Can you work these out from the model? Positions are in its coordinate system, mm. Face numbers are marked on the shaded views. A direction names the side the tool comes from. Give positions to 0.01 mm unless a question says otherwise; leave off trailing zeros. Loops run counter-clockwise (first coordinate to the right, second up) from the corner with the lowest first, then second, coordinate; pieces in that order, holes last. Notation, with made-up numbers: (25.25, -35) - (68.25, -35) arc R13 ccw to (68.25, -19) - close; hole circle Ø9 at (-27.5, 25). An arc over 180 degrees is marked (long way). Answer as a JSON object with one key per item and string values. Group by question number.
Item 1: Suppose I cut it at C-C on y = -0.75. Write out the boundary of the cut face in (x, z), and give its area (3 significant figures).
Item 2: Suppose I cut it at B-B on z = 9.5. Count the separate pieces of the cut face and the enclosed holes in it, and give its area (3 significant figures).
Item 3: Thinking about a two-plate mould opening in Y: for the marked faces 1, 2 and 3, which applies, pulls with the +Y half, pulls with the -Y half, needs draft (parallel to the pull), parting line crosses it, or undercut?
Item 4: Suppose I cut it at A-A on x = 0. Write out the boundary of the cut face in (y, z) (1 decimal).
Item 5: Which directions (+Z, -Z, +X, -X, +Y, -Y) give clear straight access to the entire face, cutting with the end or side of a thin tool? Please do the marked faces 4 and 5.
Item 6: Suppose I cut it at D-D on y = 12. Write out the boundary of the cut face in (x, z).
Item 7: Please list where these lines run through material, in increasing order: L1, parallel to Y at x = 0.25, z = 10; L2, parallel to X at y = 10.25, z = 8.25; L3, parallel to Y at x = 0, z = 8.
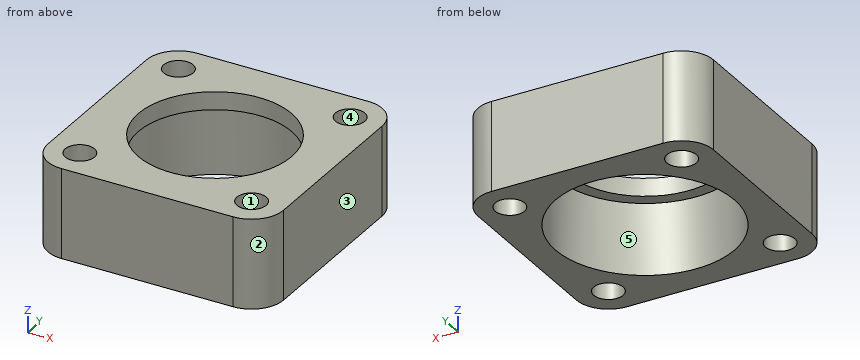
from build123d import *

# Parameters (mm, degrees)
F0_W     = 29.265608
F0_H     = 29.265608
F0_R     = 1.8288
F0_R_2   = 9.525
F1_DEPTH = 11.1125
F2_R     = 3.96875
F3_R     = 11.1125
F4_DEPTH = 8.89


with BuildPart() as f1:
    # F0 (on Top) → F1 (new body)
    with BuildSketch(Plane.XY):
        Rectangle(F0_W, F0_H)
        with Locations((-10.664054, -10.664054)):
            Circle(F0_R, mode=Mode.SUBTRACT)
        with Locations((10.664054, -10.664054)):
            Circle(F0_R, mode=Mode.SUBTRACT)
        with Locations((-10.664054, 10.664054)):
            Circle(F0_R, mode=Mode.SUBTRACT)
        Circle(F0_R_2, mode=Mode.SUBTRACT)
        with Locations((10.664054, 10.664054)):
            Circle(F0_R, mode=Mode.SUBTRACT)
    extrude(amount=F1_DEPTH)

    # F2
    f2_edges = [f1.edges().sort_by_distance(p)[0] for p in [
        (-14.632804, 14.632804, 5.55625),
        (-14.632804, -14.632804, 5.55625),
        (14.632804, -14.632804, 5.55625),
        (14.632804, 14.632804, 5.55625),
    ]]
    fillet(f2_edges, radius=F2_R)

    # F3 (on face) → F4 (cut)
    with BuildSketch(Plane(origin=(0, 0, 0), x_dir=(1, 0, 0), z_dir=(0, 0, -1))):
        Circle(F3_R)
    extrude(amount=-F4_DEPTH, mode=Mode.SUBTRACT)


solid = f1.part
Worked out:
{
 "1": {"outline": "(-14.63, 0) - (-11.09, 0) - (-11.09, 8.89) - (-9.5, 8.89) - (-9.5, 11.11) - (-14.63, 11.11) - close; (9.5, 8.89) - (11.09, 8.89) - (11.09, 0) - (14.63, 0) - (14.63, 11.11) - (9.5, 11.11) - close", "area": "85.9 mm2"},
 "2": {"separate pieces": "1", "enclosed holes": "5", "area": "516 mm2"},
 "3": {"face 1": "undercut", "face 2": "pulls with the -Y half", "face 3": "needs draft"},
 "4": {"outline": "(-14.6, 0) - (-11.1, 0) - (-11.1, 8.9) - (-9.5, 8.9) - (-9.5, 11.1) - (-14.6, 11.1) - close; (9.5, 8.9) - (11.1, 8.9) - (11.1, 0) - (14.6, 0) - (14.6, 11.1) - (9.5, 11.1) - close"},
 "5": {"face 4": "+Z, -Z", "face 5": "-Z"},
 "6": {"outline": "(-14.4, 0) - (-11.91, 0) - (-11.91, 11.11) - (-14.4, 11.11) - close; (-9.42, 0) - (9.42, 0) - (9.42, 11.11) - (-9.42, 11.11) - close; (11.91, 0) - (14.4, 0) - (14.4, 11.11) - (11.91, 11.11) - close"},
 "7": {"L1": "y = -14.63 to -9.52, 9.52 to 14.63", "L2": "x = -14.63 to -12.45, -8.88 to -4.29, 4.29 to 8.88, 12.45 to 14.63", "L3": "y = -14.63 to -11.11, 11.11 to 14.63"}
}
